Check sheet for the modelled part. Datum: model origin and axes. Units: mm. Round coordinates to 2 decimals unless told otherwise and drop trailing zeros. Write each loop counter-clockwise with the first axis right and the second up, starting at its lowest first coordinate (ties: lowest second). Pieces come first, ordered by that corner, then holes. Notation, with made-up numbers: M -2.5,41 L 30.5,41 A26 ccw 30.5,62 Z; hole C 88,-19.75 d2. An arc over 180 degrees is marked long. One line per item, written item: value.
from build123d import *

# Parameters (mm, degrees)
SKETCH1_R           = 1.5
SKETCH1_R_2         = 2.75
SKETCH1_W           = 3.2
SKETCH1_H           = 20
SKETCH1_W_2         = 20
SKETCH1_H_2         = 3.2
SKETCH1_W_3         = 80
SKETCH1_H_3         = 18
SKETCH1_W_4         = 30
SKETCH1_H_4         = 12
BOSS_EXTRUDE2_DEPTH = 3


with BuildPart() as part:
    # Sketch1 → Boss-Extrude2 (new body)
    with BuildSketch(Plane.XY):
        with BuildLine():
            Line((-35, 117.25), (-35, 57.25))
            ThreePointArc((-35, 57.25), (-36.464466094, 53.714466094), (-40, 52.25))
            Line((-40, 52.25), (-60, 52.25))
            ThreePointArc((-60, 52.25), (-63.535533906, 50.785533906), (-65, 47.25))
            Line((-65, 47.25), (-65, -79.75))
            ThreePointArc((-65, -79.75), (-64.121320344, -81.871320344), (-62, -82.75))
            Line((-62, -82.75), (62, -82.75))
            ThreePointArc((62, -82.75), (64.121320344, -81.871320344), (65, -79.75))
            Line((65, -79.75), (65, 47.25))
            ThreePointArc((65, 47.25), (63.535533906, 50.785533906), (60, 52.25))
            Line((60, 52.25), (40, 52.25))
            ThreePointArc((40, 52.25), (36.464466094, 53.714466094), (35, 57.25))
            Line((35, 57.25), (35, 117.25))
            ThreePointArc((35, 117.25), (34.414213562, 118.664213562), (33, 119.25))
            Line((33, 119.25), (-33, 119.25))
            ThreePointArc((-33, 119.25), (-34.414213562, 118.664213562), (-35, 117.25))
        make_face()
        with Locations((-20, -71.75)):
            Circle(SKETCH1_R, mode=Mode.SUBTRACT)
        with Locations((20, -71.75)):
            Circle(SKETCH1_R, mode=Mode.SUBTRACT)
        with Locations((-35, -46.75)):
            Circle(SKETCH1_R, mode=Mode.SUBTRACT)
        with Locations((35, -46.75)):
            Circle(SKETCH1_R, mode=Mode.SUBTRACT)
        with Locations((-7.865, -39.75)):
            Circle(SKETCH1_R, mode=Mode.SUBTRACT)
        with Locations((7.865, -39.75)):
            Circle(SKETCH1_R, mode=Mode.SUBTRACT)
        with Locations((-19.25, -5)):
            Circle(SKETCH1_R_2, mode=Mode.SUBTRACT)
        with Locations((19.25, -5)):
            Circle(SKETCH1_R_2, mode=Mode.SUBTRACT)
        with Locations((-50, -43.25)):
            Circle(SKETCH1_R, mode=Mode.SUBTRACT)
        with Locations((50, -43.25)):
            Circle(SKETCH1_R, mode=Mode.SUBTRACT)
        with Locations((-12.5, 108.25)):
            Circle(SKETCH1_R, mode=Mode.SUBTRACT)
        with Locations((12.5, 108.25)):
            Circle(SKETCH1_R, mode=Mode.SUBTRACT)
        with Locations((59.6, 8.25)):
            Rectangle(SKETCH1_W, SKETCH1_H, mode=Mode.SUBTRACT)
        with Locations((-59.6, 8.25)):
            Rectangle(SKETCH1_W, SKETCH1_H, mode=Mode.SUBTRACT)
        with Locations((0, 54.75)):
            Rectangle(SKETCH1_W_2, SKETCH1_H_2, mode=Mode.SUBTRACT)
        with Locations((0, -58.75)):
            Rectangle(SKETCH1_W_3, SKETCH1_H_3, mode=Mode.SUBTRACT)
        with Locations((0, -26.75)):
            Rectangle(SKETCH1_W_4, SKETCH1_H_4, mode=Mode.SUBTRACT)
        with Locations((0, 114.75)):
            Rectangle(SKETCH1_W_2, SKETCH1_H_2, mode=Mode.SUBTRACT)
    extrude(amount=BOSS_EXTRUDE2_DEPTH)


solid = part.part
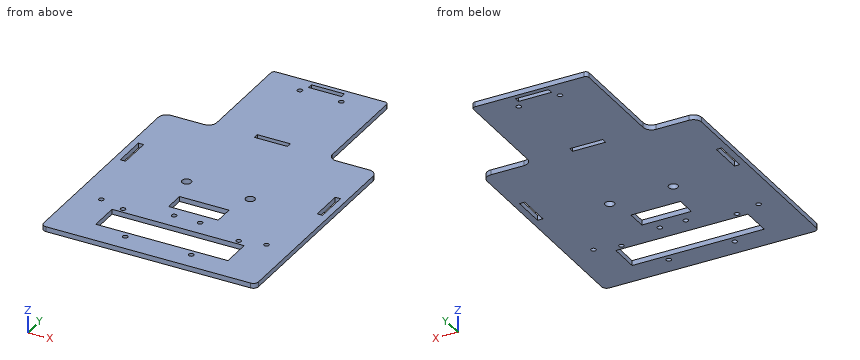
Q1. Sectioned sample at D-D on y = 92.5. Enter the section's corners in (x, z).
Completed:
outline: M -35,0 L 35,0 L 35,3 L -35,3 Z
Q2. Sectioned sample at C-C on z = 1.3. State how many separate pieces and enclosed holes the cut face has, and give its area (3 significant figures).
Completed:
separate pieces: 1
enclosed holes: 18
area: 20,100 mm^2
Q3. Scan lines: line 1 (Y direction, x = 12.5, z = 2.1); line 2 (Y direction, x = 0.5, z = 1.05); line 3 (X direction, y = -71.75, z = 0.8). Record each from-to range of solid material in increasing order. Write a range as [from, to].
Completed:
line 1: [-82.75, -67.75], [-49.75, -32.75], [-20.75, 106.75], [109.75, 119.25]
line 2: [-82.75, -67.75], [-49.75, -32.75], [-20.75, 53.15], [56.35, 113.15], [116.35, 119.25]
line 3: [-65, -21.5], [-18.5, 18.5], [21.5, 65]
Q4. Sectioned sample at B-B on x = 29. Enter the section's corners in (y, z).
Completed:
outline: M -82.75,0 L -67.75,0 L -67.75,3 L -82.75,3 Z; M -49.75,0 L 119.25,0 L 119.25,3 L -49.75,3 Z
Q5. Depth check by flat-ended pin: P1, Ø1.5, axis at x = 59, z = 1.5, coming from the +Y side; P2, Ø1.5, axis at y = 114, z = 1.5, coming from the +X side. Enter the tip coordinate at first touch or a pass-through.
Completed:
P1: y = 52.25
P2: x = 35
Q6. Sectioned sample at A-A on y = 14. Enter the section's corners in (x, z).
Completed:
outline: M -65,0 L -61.2,0 L -61.2,3 L -65,3 Z; M -58,0 L 58,0 L 58,3 L -58,3 Z; M 61.2,0 L 65,0 L 65,3 L 61.2,3 Z
